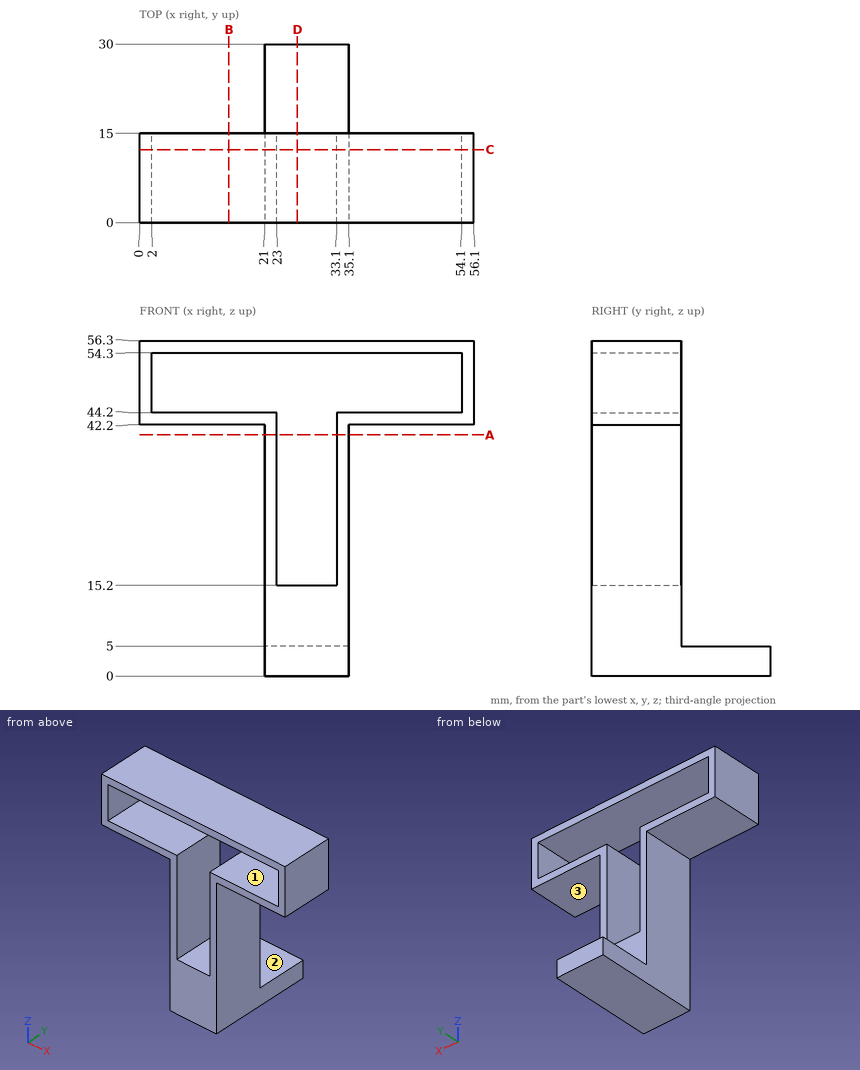
Here's the drawing with two shaded views (mm, measured from the low corner). I have some questions. A direction names the side the tool comes from. Round coordinates to 2 decimals unless told otherwise and drop trailing zeros. Loops run counter-clockwise (first coordinate to the right, second up) from the corner with the lowest first, then second, coordinate; pieces in that order, holes last.
Item 1: Suppose I cut it at A-A, the plane z = 40.5. Write out the boundary of the cut face in (x, y).
Item 2: Suppose I cut it at B-B, the plane x = 15. Write out the boundary of the cut face in (y, z).
Item 3: Suppose I cut it at D-D, the plane x = 26.5. Write out the boundary of the cut face in (y, z), then the cut area to 3 significant figures.
Item 4: Will these pins go through, and if not, where does the flat tip stop? pin 1 Ø16.5 at (y, z) = (10, 33.5) entering from +X; pin 2 Ø4.5 at (y, z) = (7, 23.5) entering from -X; pin 3 Ø4 at (x, y) = (10, 9) entering from -Z.
Item 5: Suppose I cut it at C-C, the plane y = 12.25. Write out the boundary of the cut face in (x, z), then the cut area to 3 significant figures.
Item 6: Please list where these lines run through material, in increasing order: L1, parallel to Z at x = 33.5, y = 14.5; L2, parallel to X at y = 7.75, z = 18; L3, parallel to X at y = 10.5, z = 52.
Item 7: Which directions (+Z, -Z, +X, -X, +Y, -Y) give clear straight access to the entire face, cutting with the end or side of a thin tool? Please do the marked faces 1, 2 and 3.
Reported:
1. outline: (21, 0) - (23, 0) - (23, 15) - (21, 15) - close; (33.1, 0) - (35.1, 0) - (35.1, 15) - (33.1, 15) - close
2. outline: (0, 42.2) - (15, 42.2) - (15, 44.2) - (0, 44.2) - close; (0, 54.3) - (15, 54.3) - (15, 56.3) - (0, 56.3) - close
3. outline: (0, 0) - (30, 0) - (30, 5) - (15, 5) - (15, 15.2) - (0, 15.2) - close; (0, 54.3) - (15, 54.3) - (15, 56.3) - (0, 56.3) - close
3. area: 333 mm2
4. pin 1: stops at x = 35.1
4. pin 2: stops at x = 21
4. pin 3: stops at z = 42.2
5. outline: (0, 42.2) - (21, 42.2) - (21, 0) - (35.1, 0) - (35.1, 42.2) - (56.1, 42.2) - (56.1, 56.3) - (0, 56.3) - close; hole (2, 44.2) - (23, 44.2) - (23, 15.2) - (33.1, 15.2) - (33.1, 44.2) - (54.1, 44.2) - (54.1, 54.3) - (2, 54.3) - close
5. area: 567 mm2
6. L1: z = 0 to 44.2, 54.3 to 56.3
6. L2: x = 21 to 23, 33.1 to 35.1
6. L3: x = 0 to 2, 54.1 to 56.1
7. face 1: +Y, -Y
7. face 2: +Z, +X, -X, +Y
7. face 3: -Z, +X, +Y, -Y
